from build123d import *

# Parameters (mm, degrees)
F0_R           = 25
F0_R_2         = 20
F4_DEPTH       = 80
F5_R           = 1.5
F6_DEPTH       = 84
F6_DEPTH_BACK  = 4
F8_DEPTH       = 35.3563390593
F8_DEPTH_BACK  = 25
F10_DEPTH      = 35.3563390593
F10_DEPTH_BACK = 25
F13_R          = 1.5
F14_DEPTH      = 35
F14_DEPTH_BACK = 35
F11_W          = 30.2
F11_H          = 4
F11_R          = 3.5
F15_DEPTH      = 4.1
F15_DEPTH_BACK = 4.1


with BuildPart() as f4:
    # F0 (on Front) → F4 (new body)
    with BuildSketch(Plane.XZ):
        Circle(F0_R)
        Circle(F0_R_2, mode=Mode.SUBTRACT)
    extrude(amount=F4_DEPTH)

    # F5 (on Front) → F6 (cut, two sides)
    with BuildSketch(Plane.XZ) as f6_sk:
        with Locations((0, 22.5)):
            Circle(F5_R)
        with Locations((0, -22.5)):
            Circle(F5_R)
        with Locations((-22.5, 0)):
            Circle(F5_R)
        with Locations((22.5, 0)):
            Circle(F5_R)
    extrude(amount=F6_DEPTH, mode=Mode.SUBTRACT)
    extrude(f6_sk.sketch, amount=-F6_DEPTH_BACK, mode=Mode.SUBTRACT)

    # F7 (on line) → F8 (cut, two sides)
    with BuildSketch(Plane(origin=(0, 0, 0), x_dir=(0.7071067812, 0, 0.7071067812), z_dir=(0.7071067812, 0, -0.7071067812))) as f8_sk:
        Polygon((-11.31, 40), (0, 8), (11.31, 40), (0, 72), align=None)
    extrude(amount=-F8_DEPTH, mode=Mode.SUBTRACT)
    extrude(f8_sk.sketch, amount=F8_DEPTH_BACK, mode=Mode.SUBTRACT)

    # F9 (on line) → F10 (cut, two sides)
    with BuildSketch(Plane(origin=(0, 0, 0), x_dir=(0.7071067812, 0, -0.7071067812), z_dir=(-0.7071067812, 0, -0.7071067812))) as f10_sk:
        Polygon((-11.31, 40), (0, 8), (11.31, 40), (0, 72), align=None)
    extrude(amount=-F10_DEPTH, mode=Mode.SUBTRACT)
    extrude(f10_sk.sketch, amount=F10_DEPTH_BACK, mode=Mode.SUBTRACT)

    # F13 (on offset) → F14 (join, two sides)
    with BuildSketch(Plane.XZ.offset(40)) as f14_sk:
        with Locations((0, 22.5)):
            Circle(F13_R)
        with Locations((0, -22.5)):
            Circle(F13_R)
        with Locations((22.5, 0)):
            Circle(F13_R)
        with Locations((-22.5, 0)):
            Circle(F13_R)
    extrude(amount=F14_DEPTH)
    extrude(f14_sk.sketch, amount=-F14_DEPTH_BACK)

    # F11 (on Right) → F15 (cut, two sides)
    with BuildSketch(Plane.YZ) as f15_sk:
        with Locations((-39.9, -26)):
            Rectangle(F11_W, F11_H)
        with BuildLine():
            Line((-24.8, -28), (-55, -28))
            Line((-55, -28), (-53.4000304969, -28.5403946475))
            ThreePointArc((-53.4000304969, -28.5403946475), (-50.9379901825, -30.3620036381), (-50, -33.2774926609))
            Line((-50, -33.2774926609), (-50, -43.9965311409))
            ThreePointArc((-50, -43.9965311409), (-48.5355339059, -47.5320650468), (-45, -48.9965311409))
            Line((-45, -48.9965311409), (-35, -48.9965311409))
            ThreePointArc((-35, -48.9965311409), (-31.4644660941, -47.5320650468), (-30, -43.9965311409))
            Line((-30, -43.9965311409), (-30, -33.1293155523))
            ThreePointArc((-30, -33.1293155523), (-28.853919359, -29.9438319824), (-25.9410777703, -28.2186768331))
            Line((-25.9410777703, -28.2186768331), (-24.8, -28))
        make_face()
        with Locations((-40, -38.9965311409)):
            Circle(F11_R, mode=Mode.SUBTRACT)
    extrude(amount=F15_DEPTH, mode=Mode.SUBTRACT)
    extrude(f15_sk.sketch, amount=-F15_DEPTH_BACK, mode=Mode.SUBTRACT)


solid = f4.part
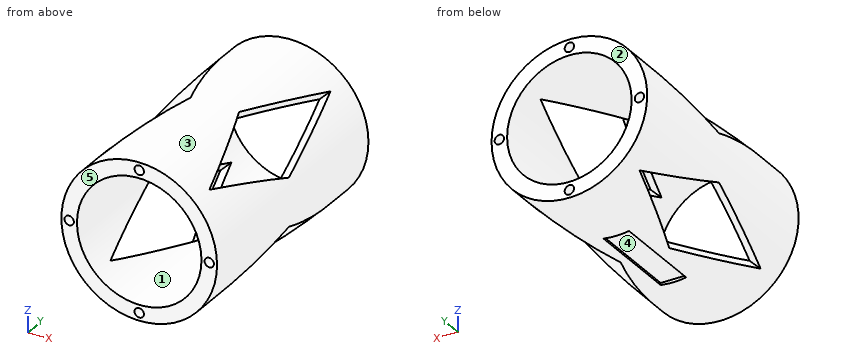
The model under review builds one solid part; all positions refer to its coordinate system, in mm. Face numbers are marked on the shaded views. A direction names the side the tool comes from. Give positions to 0.01 mm unless a question says otherwise; leave off trailing zeros. Order: outer loops, then holes, each group sorted by start corner. A loop starts at its lowest first (then second) coordinate and runs counter-clockwise, first axis right, second up. Notation, with made-up numbers: M -11,87.5 L 27,87.5 A32 ccw 27,125.5 Z; hole C -25.5,33.25 d11. An arc over 180 degrees is marked long. Answer in a Markdown table with one row per item. Add a question column.
1. Machinability: for the marked faces 4 and 5, which of the approach directions +Z, -Z, +X, -X, +Y, -Y give a long, thin tool a straight path to every point of the face, cutting with its end or side? Answer none if there is none.
2. Add section A-A on x = 0. State the section outline as (y, z) points, plus the area to 3 significant figures.
3. Mouldability with a two-part tool opening along X and no side actions: class the marked faces 1, 2 and 3 as released by +X, released by -X, zero draft, split by the parting line, or undercut.
4. Add section C-C on z = 13. State the section outline as (x, y) points, plus the area to 3 significant figures.
5. To check wall thickness, follow line 1 along Z through (x, y) = (0, -78.15); line 2 along Z through (x, y) = (-0.5, -25) (3 decimals); line 3 along Z through (x, y) = (0, -13.5). State the ranges of each line that lie inside material, in increasing order.
6. Add section B-B on z = 0. State the section outline as (x, y) points.
7. For pin 1 Ø0.9 at (x, z) = (0.5, 22) entering from +Y; pin 2 Ø1 at (y, z) = (-29, -16.5) entering from +X; pin 3 Ø1.5 at (x, y) = (6.5, -9.5) entering from -Z; pin 4 Ø5 at (x, y) = (-9.5, -25.5) entering from +Z, all flat-tipped, find the tip position at first contact; note any pin that passes through.
8. Add section D-D on y = -60.5. State the section outline as (x, z) points.
The answers:
| question | item | result |
|---|---|---|
| 1 | face 4 | -Z |
| 1 | face 5 | +Z, -Z, +X, -X, -Y |
| 2 | outline | M -80,-25 L -55,-25 L -55,-24 L -24.8,-24 L -24.8,-25 L 0,-25 L 0,-24 L -5,-24 L -5,-21 L 0,-21 L 0,-20 L -80,-20 L -80,-21 L -75,-21 L -75,-24 L -80,-24 Z; M -80,20 L 0,20 L 0,21 L -5,21 L -5,24 L 0,24 L 0,25 L -80,25 L -80,24 L -75,24 L -75,21 L -80,21 Z |
| 2 | area | 710 mm2 |
| 3 | face 1 | undercut |
| 3 | face 2 | zero draft |
| 3 | face 3 | split by the parting line |
| 4 | outline | M -21.35,-80 L -15.2,-80 L -15.2,-67.6 L -21.35,-55.29 Z; M -21.35,-24.71 L -15.2,-12.4 L -15.2,0 L -21.35,0 Z; M 15.2,-80 L 21.35,-80 L 21.35,-55.29 L 15.2,-67.6 Z; M 15.2,-12.4 L 21.35,-24.71 L 21.35,0 L 15.2,0 Z |
| 4 | area | 457 mm2 |
| 5 | line 1 | -25 to -24, -21 to -20, 20 to 21, 24 to 25 |
| 5 | line 2 | -24 to -19.994, 19.994 to 24.995 |
| 5 | line 3 | -25 to -20, 20 to 25 |
| 6 | outline | M -25,-80 L -24,-80 L -24,-75 L -21,-75 L -21,-80 L -20,-80 L -20,0 L -21,0 L -21,-5 L -24,-5 L -24,0 L -25,0 Z; M 20,-80 L 21,-80 L 21,-75 L 24,-75 L 24,-80 L 25,-80 L 25,0 L 24,0 L 24,-5 L 21,-5 L 21,0 L 20,0 Z |
| 7 | pin 1 | y = -5 |
| 7 | pin 2 | through |
| 7 | pin 3 | z = -24.33 |
| 7 | pin 4 | z = 24 |
| 8 | outline | M -20.32,-14.57 L -16.72,-10.97 A20 cw -16.72,10.97 L -20.32,14.57 A25 ccw Z; M -14.57,-20.32 A25 ccw 14.57,-20.32 L 10.97,-16.72 A20 cw -10.97,-16.72 Z; M -14.57,20.32 L -10.97,16.72 A20 cw 10.97,16.72 L 14.57,20.32 A25 ccw Z; M 16.72,-10.97 L 20.32,-14.57 A25 ccw 20.32,14.57 L 16.72,10.97 A20 cw Z |
